Geometry: final body of the model. Coordinates: model frame, mm. Face numbers are marked on the shaded views. A direction names the side the tool comes from. Round coordinates to 2 decimals unless told otherwise and drop trailing zeros. Loops run counter-clockwise (first coordinate to the right, second up) from the corner with the lowest first, then second, coordinate; pieces in that order, holes last. Notation, with made-up numbers: (-7, 82) -> (36, 82) arc R28 cw to (36, 110) -> close; hole circle Ø4 at (39.25, 77.5). An arc over 180 degrees is marked (long way). Answer in a Markdown table with one row per item.
```python
from build123d import *

# Parameters (mm, degrees)
SKETCH1_R             = 7.9629
BOSS_EXTRUDE1_DEPTH   = 6.35
F_6_32_TAPPED_HOLE1_D = 2.7051


with BuildPart() as part:
    # Sketch1 → Boss-Extrude1 (new body)
    with BuildSketch(Plane.XY.offset(7.874)):
        with BuildLine():
            ThreePointArc((8.047909304, 6.74848607), (6.173449726, 8.49702459), (3.931250908, 9.739413469))
            ThreePointArc((3.931250908, 9.739413469), (3.309450684, 10.277458281), (3.147581267, 11.08363818))
            ThreePointArc((3.147581267, 11.08363818), (0, 14.675), (-3.147581267, 11.08363818))
            ThreePointArc((-3.147581267, 11.08363818), (-3.309450684, 10.277458281), (-3.931250908, 9.739413469))
            ThreePointArc((-3.931250908, 9.739413469), (-6.173449726, 8.49702459), (-8.047909304, 6.74848607))
            ThreePointArc((-8.047909304, 6.74848607), (-8.751767166, 6.323383906), (-9.568510213, 6.418560232))
            ThreePointArc((-9.568510213, 6.418560232), (-13.956754377, 4.534824392), (-11.513822419, 0.431504882))
            ThreePointArc((-11.513822419, 0.431504882), (-10.797120172, 0.028434629), (-10.477555984, -0.729197516))
            ThreePointArc((-10.477555984, -0.729197516), (-9.988851485, -3.24557459), (-8.905132396, -5.568619705))
            ThreePointArc((-8.905132396, -5.568619705), (-8.718340254, -6.369392103), (-9.061245801, -7.116749798))
            ThreePointArc((-9.061245801, -7.116749798), (-8.625748577, -11.872324392), (-3.968352328, -10.816953497))
            ThreePointArc((-3.968352328, -10.816953497), (-3.363536563, -10.259884713), (-2.544234809, -10.190082318))
            ThreePointArc((-2.544234809, -10.190082318), (0, -10.5029), (2.544234809, -10.190082318))
            ThreePointArc((2.544234809, -10.190082318), (3.363536563, -10.259884713), (3.968352328, -10.816953497))
            ThreePointArc((3.968352328, -10.816953497), (8.625748577, -11.872324392), (9.061245801, -7.116749798))
            ThreePointArc((9.061245801, -7.116749798), (8.718340254, -6.369392103), (8.905132396, -5.568619705))
            ThreePointArc((8.905132396, -5.568619705), (9.988851485, -3.24557459), (10.477555984, -0.729197516))
            ThreePointArc((10.477555984, -0.729197516), (10.797120172, 0.028434629), (11.513822419, 0.431504882))
            ThreePointArc((11.513822419, 0.431504882), (13.956754377, 4.534824392), (9.568510213, 6.418560232))
            ThreePointArc((9.568510213, 6.418560232), (8.751767166, 6.323383906), (8.047909304, 6.74848607))
        make_face()
        Circle(SKETCH1_R, mode=Mode.SUBTRACT)
    extrude(amount=BOSS_EXTRUDE1_DEPTH)

    # #6-32 Tapped Hole1 (through all)
    with Locations(Plane.XY.offset(14.224)):
        with Locations((-10.937149937, 3.553695435), (0, 11.5), (10.937149937, 3.553695435), (6.759530401, -9.303695435), (-6.759530401, -9.303695435)):
            Hole(F_6_32_TAPPED_HOLE1_D / 2)


solid = part.part
```
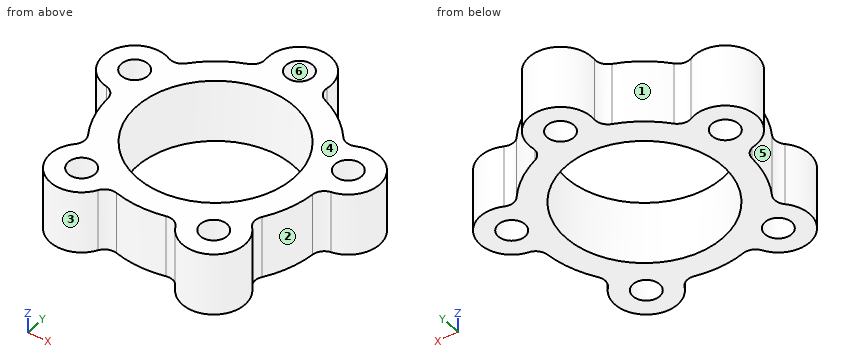
Item 1: Ray query, L1, parallel to X at y = 3.75, z = 9.25; L2, parallel to X at y = 2.5, z = 9; L3, parallel to Y at x = 6.5, z = 10. Return the intervals inside material, ascending.
Ans:
| item | result |
|---|---|
| L1 | -14.11 to -12.28, -9.6 to -7.02, 7.02 to 9.6, 12.28 to 14.11 |
| L2 | -13.93 to -11.79, -10.09 to -7.56, 7.56 to 10.09, 11.79 to 13.93 |
| L3 | -12.47 to -10.63, -7.98 to -4.6, 4.6 to 8.25 |
Item 2: Section query A-A, the plane x = 0. Output: boundary loops of the cut face in (y, z) (3 decimals), and give its area (3 significant figures).
Ans:
| item | result |
|---|---|
| outline | (-10.503, 7.874) -> (-7.963, 7.874) -> (-7.963, 14.224) -> (-10.503, 14.224) -> close; (7.963, 7.874) -> (10.147, 7.874) -> (10.147, 14.224) -> (7.963, 14.224) -> close; (12.853, 7.874) -> (14.675, 7.874) -> (14.675, 14.224) -> (12.853, 14.224) -> close |
| area | 41.6 mm2 |
Item 3: Section query D-D, the plane z = 13.25. State how many separate pieces and enclosed holes the cut face has, and give its area (3 significant figures).
Ans:
| item | result |
|---|---|
| separate pieces | 1 |
| enclosed holes | 6 |
| area | 236 mm2 |
Item 4: Section query B-B, the plane y = 11.5. Output: boundary loops of the cut face in (x, z) (3 decimals).
Ans:
| item | result |
|---|---|
| outline | (-3.175, 7.874) -> (-1.353, 7.874) -> (-1.353, 14.224) -> (-3.175, 14.224) -> close; (1.353, 7.874) -> (3.175, 7.874) -> (3.175, 14.224) -> (1.353, 14.224) -> close |
Item 5: Set-up query: the marked faces 5 and 6. Return all of +Z, -Z, +X, -X, +Y, -Y with unobstructed straight access to the full face (end or side cutting, diameter ignored); none if empty.
Ans:
| item | result |
|---|---|
| face 5 | +Z, -Z, -X |
| face 6 | +Z, -Z |
Item 6: Mould query, pull axis X, two halves, no side actions, for the marked faces 1, 2, 3 and 4. Classes: released by +X, released by -X, zero draft, split by the parting line, or undercut.
Ans:
| item | result |
|---|---|
| face 1 | released by -X |
| face 2 | released by +X |
| face 3 | undercut |
| face 4 | zero draft |
Item 7: Section query C-C, the plane x = -4.75. Output: boundary loops of the cut face in (y, z).
Ans:
| item | result |
|---|---|
| outline | (-11.76, 7.87) -> (-6.39, 7.87) -> (-6.39, 14.22) -> (-11.76, 14.22) -> close; (6.39, 7.87) -> (9.37, 7.87) -> (9.37, 14.22) -> (6.39, 14.22) -> close |
